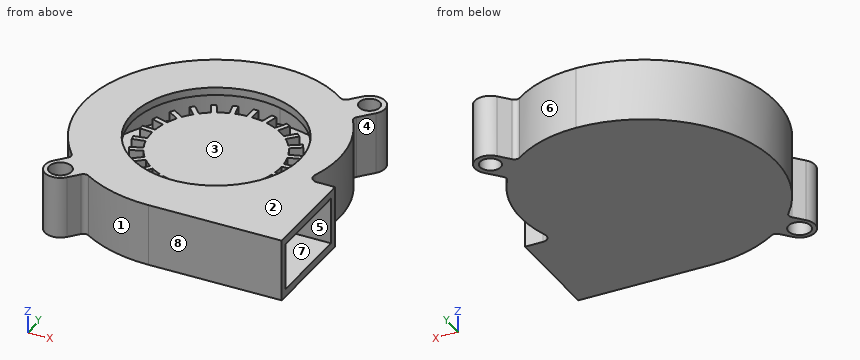
from build123d import *

# Parameters (mm, degrees)
BOSS_EXTRUDE1_DEPTH = 12
CUT_EXTRUDE2_DEPTH  = 28.5
SHELL1_T            = -1.5
SKETCH2_R           = 16.25
CUT_EXTRUDE1_DEPTH  = 3.76
SKETCH3_R           = 12.5
BOSS_EXTRUDE2_DEPTH = 7.76
BOSS_EXTRUDE3_DEPTH = 7.76
CIRPATTERN1_COUNT   = 25
FILLET1_R           = 1.5
SKETCH6_R           = 2.15
BOSS_EXTRUDE4_DEPTH = 12
FILLET2_R           = 1
SKETCH7_R           = 2
BOSS_EXTRUDE5_DEPTH = 12
FILLET3_R           = 1


with BuildPart() as part:
    # Sketch1 → Boss-Extrude1 (new body)
    with BuildSketch(Plane.XY):
        with BuildLine():
            Line((0, -25.5), (25.8, -25.5))
            Line((25.8, -25.5), (25.8, -5.5))
            Line((25.8, -5.5), (24.899799196, -5.5))
            ThreePointArc((24.899799196, -5.5), (-15.968719423, 19.880895352), (0, -25.5))
        make_face()
    extrude(amount=BOSS_EXTRUDE1_DEPTH)

    # Sketch5 → Cut-Extrude2 (cut)
    with BuildSketch(Plane.XY.offset(12)):
        with BuildLine():
            Line((24.899799196, -5.5), (20.18266583, -5.5))
            ThreePointArc((20.18266583, -5.5), (18.495540003, 15.471590427), (0, 25.5))
            ThreePointArc((0, 25.5), (19.880895352, 15.968719423), (24.899799196, -5.5))
        make_face()
    extrude(amount=-CUT_EXTRUDE2_DEPTH, mode=Mode.SUBTRACT)

    # Shell1
    shell1_openings = [part.faces().sort_by_distance(p)[0] for p in [
        (25.8, -15.5, 6),
    ]]
    offset(amount=SHELL1_T, openings=shell1_openings, kind=Kind.INTERSECTION)

    # Sketch2 → Cut-Extrude1 (cut)
    with BuildSketch(Plane.XY.offset(12)):
        Circle(SKETCH2_R)
    extrude(amount=-CUT_EXTRUDE1_DEPTH, mode=Mode.SUBTRACT)

    # Sketch3 → Boss-Extrude2 (add)
    with BuildSketch(Plane.XY.offset(1.5)):
        Circle(SKETCH3_R)
    extrude(amount=BOSS_EXTRUDE2_DEPTH)

    # Sketch4 → Boss-Extrude3 (add)
    with BuildSketch(Plane.XY.offset(1.5)):
        with BuildLine():
            Line((-0.5, 12.489995997), (-0.5, 14.989995997))
            Line((-0.5, 14.989995997), (0.5, 14.989995997))
            Line((0.5, 14.989995997), (0.5, 12.489995997))
            ThreePointArc((0.5, 12.489995997), (0, 12.5), (-0.5, 12.489995997))
        make_face()
    boss_extrude3 = extrude(amount=BOSS_EXTRUDE3_DEPTH)

    # CirPattern1: Boss-Extrude3 ×25 about axis
    cirpattern1_axis = Axis((0, 0, 0), (0, 0, 1))
    for i in range(1, CIRPATTERN1_COUNT):
        add(boss_extrude3.rotate(cirpattern1_axis, i * 360 / CIRPATTERN1_COUNT))

    # Fillet1
    fillet1_edges = [part.edges().sort_by_distance(p)[0] for p in [
        (20.18266583, -5.5, 6),
    ]]
    fillet(fillet1_edges, radius=FILLET1_R)

    # Sketch6 → Boss-Extrude4 (add)
    with BuildSketch(Plane.XY.offset(12)):
        with BuildLine():
            Line((-18.877455455, -17.143269104), (-21.173662056, -19.784752634))
            ThreePointArc((-21.173662056, -19.784752634), (-20.877710402, -24.017058462), (-16.645404575, -23.721106808))
            Line((-16.645404575, -23.721106808), (-14.349197973, -21.079623278))
            ThreePointArc((-14.349197973, -21.079623278), (-16.729505239, -19.245094296), (-18.877455455, -17.143269104))
        make_face()
        with Locations((-18.909533315, -21.752929721)):
            Circle(SKETCH6_R, mode=Mode.SUBTRACT)
    extrude(amount=-BOSS_EXTRUDE4_DEPTH)

    # Fillet2
    fillet2_edges = [part.edges().sort_by_distance(p)[0] for p in [
        (-14.349197973, -21.079623278, 6),
        (-18.877455455, -17.143269104, 6),
    ]]
    fillet(fillet2_edges, radius=FILLET2_R)

    # Sketch7 → Boss-Extrude5 (add)
    with BuildSketch(Plane.XY.offset(12)):
        with BuildLine():
            Line((13.905047135, 20.568686185), (16.365268494, 23.398847111))
            ThreePointArc((16.365268494, 23.398847111), (20.597574322, 23.694798765), (20.893525975, 19.462492937))
            Line((20.893525975, 19.462492937), (18.02598514, 16.163764554))
            ThreePointArc((18.02598514, 16.163764554), (16.116716142, 18.507677567), (13.905047135, 20.568686185))
        make_face()
        with Locations((18.629397235, 21.430670024)):
            Circle(SKETCH7_R, mode=Mode.SUBTRACT)
    extrude(amount=-BOSS_EXTRUDE5_DEPTH)

    # Fillet3
    fillet3_edges = [part.edges().sort_by_distance(p)[0] for p in [
        (13.905047135, 20.568686185, 6),
        (18.02598514, 16.163764554, 6),
    ]]
    fillet(fillet3_edges, radius=FILLET3_R)


solid = part.part
The listing builds one solid part. Answer for the finished solid, in the listing's coordinates (mm). Face numbers are marked on the shaded views. A direction names the side the tool comes from. Coordinates: 2 decimals unless noted, no trailing zeros. Put each result on its own line as item: value. Start each with the question number.
1. Flat-ended cylindrical pins translate along their axes: P1, Ø1.3, axis at y = 13, z = 7, coming from the +X side; P2, Ø1.3, axis at y = 14, z = 6.5, coming from the -X side; P3, Ø5, axis at y = 1.5, z = 8, coming from the +X side. Find the tip coordinate at first contact, or state that the pin passes through.
2. Consider line 1 (Z direction, x = 5, y = 22.5); line 2 (Y direction, x = 18, z = 7); line 3 (X direction, y = -6.5, z = 7). Determine where each line is inside the solid, lowest interval first. Write a range as from..to.
3. For a pull along Y with two mould halves and no side action, classify the marked faces 1, 2 and 3 as pulls with the +Y half, pulls with the -Y half, needs draft (parallel to the pull), parting line crosses it, or undercut.
4. Which of the six approach directions +Z, -Z, +X, -X, +Y, -Y give full straight-line access (tool end or side, diameter ignored) to the marked faces 4, 5, 6, 7 and 8?
5. A cutting plane is placed at A-A on z = 4.5. Count the separate pieces of the cut face and the enclosed holes in it, then the cut area to 3 significant figures.
Resolved:
1. P1: stops at x = 20.19
1. P2: stops at x = -21.73
1. P3: stops at x = 22.07
2. line 1: z = 0..1.5, 10.5..12
2. line 2: y = -25.5..-24, -7..-6.53, 13.39..19.53, 23.33..24.36
2. line 3: x = -24.66..-23.1, -13.51..-12.64, -10.68..10.68, 12.64..13.51, 18.01..25.8
3. face 1: pulls with the -Y half
3. face 2: needs draft
3. face 3: undercut
4. face 4: +Z, -Z, +X
4. face 5: +X
4. face 6: +Z, -Z, +Y
4. face 7: none
4. face 8: +Z, -Z, +X, -X, -Y
5. separate pieces: 2
5. enclosed holes: 2
5. area: 831 mm2
